The figure shows three views and two pictorial views of one solid part (mm, origin at its lowest corner). Answer the questions. Coordinates: 2 decimals unless noted, no trailing zeros. Write each loop counter-clockwise with the first axis right and the second up, starting at its lowest first coordinate (ties: lowest second). Pieces come first, ordered by that corner, then holes.
Item 1: Section A-A (x = 30) is taken. Give the vertices of the cut face in (y, z), then the cut area to 3 significant figures.
Item 2: Section D-D (x = 52) is taken. Give the vertices of the cut face in (y, z).
Item 3: Section B-B (z = 5) is taken. Give the vertices of the cut face in (x, y), then the cut area to 3 significant figures.
Item 4: Each of these flat-tipped pins is pushed along its axis until it touches: P1, Ø4, axis at x = 8.35, z = 42.5, coming from the +Y side; P2, Ø4, axis at y = 5, z = 43.5, coming from the -X side; P3, Ø1.5, axis at x = 46, y = 2, coming from the +Z side (1 decimal). Where does it stop, or does it pass through?
Item 5: Section C-C (z = 42.5) is taken. Give the vertices of the cut face in (x, y), then the cut area to 3 significant figures.
Item 6: Straight lines are drawn through the part: probe 1 along Z at (x, y) = (30, 6.9); probe 2 along X at (y, z) = (6.5, 45); probe 3 along X at (y, z) = (2.85, 42.5). For each, find the intervals that lie inside material, in ascending order.
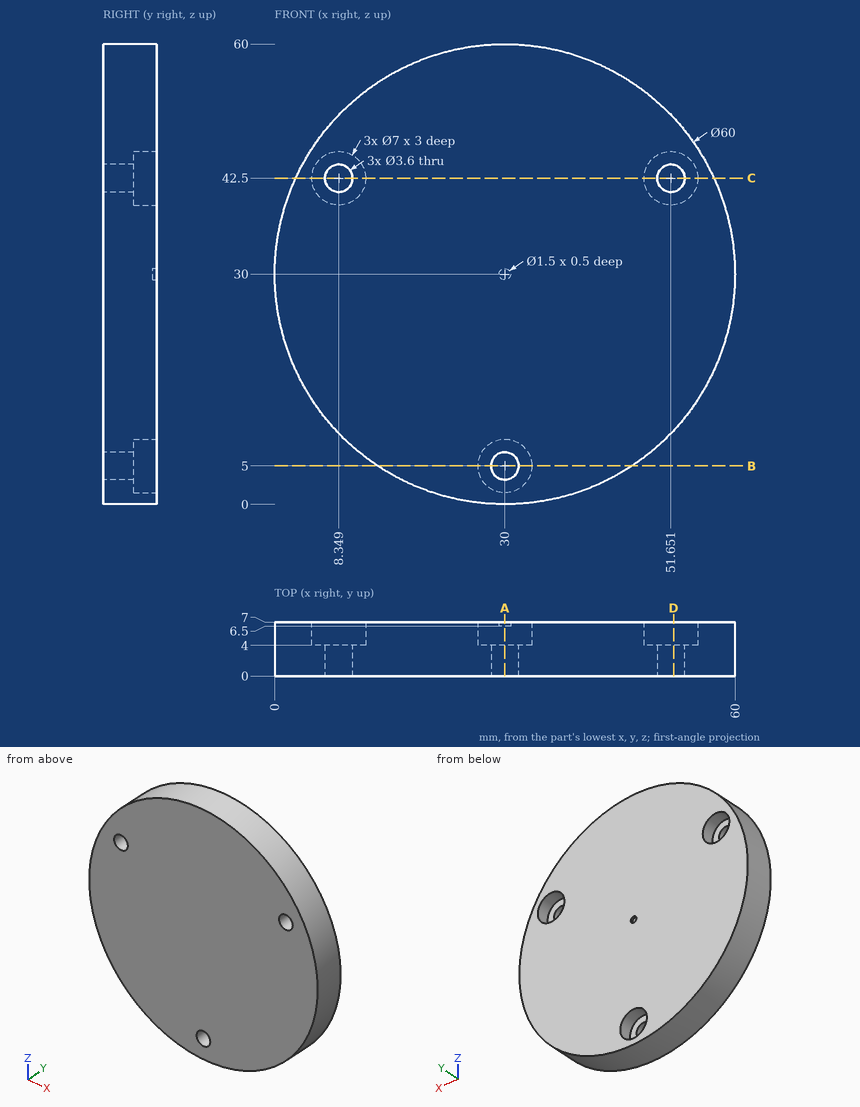
Established:
1. outline: (0, 0) - (7, 0) - (7, 1.5) - (4, 1.5) - (4, 3.2) - (0, 3.2) - close; (0, 6.8) - (4, 6.8) - (4, 8.5) - (7, 8.5) - (7, 29.25) - (6.5, 29.25) - (6.5, 30.75) - (7, 30.75) - (7, 60) - (0, 60) - close
1. area: 384 mm2
2. outline: (0, 9.6) - (7, 9.6) - (7, 39.02) - (4, 39.02) - (4, 40.73) - (0, 40.73) - close; (0, 44.27) - (4, 44.27) - (4, 45.98) - (7, 45.98) - (7, 50.4) - (0, 50.4) - close
3. outline: (13.42, 0) - (28.2, 0) - (28.2, 4) - (26.5, 4) - (26.5, 7) - (13.42, 7) - close; (31.8, 0) - (46.58, 0) - (46.58, 7) - (33.5, 7) - (33.5, 4) - (31.8, 4) - close
3. area: 197 mm2
4. P1: stops at y = 4
4. P2: stops at x = 2.29
4. P3: stops at z = 55.8
5. outline: (2.73, 0) - (6.55, 0) - (6.55, 4) - (4.85, 4) - (4.85, 7) - (2.73, 7) - close; (10.15, 0) - (49.85, 0) - (49.85, 4) - (48.15, 4) - (48.15, 7) - (11.85, 7) - (11.85, 4) - (10.15, 4) - close; (53.45, 0) - (57.27, 0) - (57.27, 7) - (55.15, 7) - (55.15, 4) - (53.45, 4) - close
5. area: 311 mm2
6. probe 1: z = 0 to 1.5, 8.5 to 29.25, 30.75 to 60
6. probe 2: x = 4.02 to 5.9, 10.8 to 49.2, 54.1 to 55.98
6. probe 3: x = 2.73 to 6.55, 10.15 to 49.85, 53.45 to 57.27
